Model file for the job. Use its own axes, mm. Face numbers are marked on the shaded views. A direction names the side the tool comes from. Give positions to 0.01 mm unless a question says otherwise; leave off trailing zeros. Loops run counter-clockwise (first coordinate to the right, second up) from the corner with the lowest first, then second, coordinate; pieces in that order, holes last. Notation, with made-up numbers: (-24.5, 78) -> (7.5, 78) arc R18 ccw to (7.5, 108) -> close; hole circle Ø10 at (-14, -29.75). An arc over 180 degrees is marked (long way). Use CSV: the item, a comma, the result in double quotes. Start each with the question number.
(1) Pull direction Y, two halves, no side cores. Call the marked faces 3, 4 and 5: pulls with the +Y half, pulls with the -Y half, needs draft (parallel to the pull), parting line crosses it, or undercut.
(2) Drill centre lines: probe 1 along X at (y, z) = (16, 2.25); probe 2 along X at (y, z) = (35.5, 6.75); probe 3 along Z at (x, y) = (23.5, 47). Where is each one in solid material? Low to high.
(3) Cut at B-B on y = 7. Write the cut outline in (x, z), then the cut area to 3 significant figures.
(4) Flat gauge pins, fed straight in: pin 1 (1.6 mm diameter, centred on x = 50, z = 4, fed in from +Y); pin 2 (0.8 mm diameter, centred on x = -18, z = 5.5, fed in from +Y); pin 3 (1.5 mm diameter, centred on x = 10.5, z = 6, fed in from -Y); pin 4 (1.2 mm diameter, centred on x = 35, y = 39.5, fed in from +Z). Where does each tip first touch, or does it go through?
(5) 3-axis set-ups, long thin cutter, end or side, ignore diameter. For the marked faces 1 and 2: which of +Z, -Z, +X, -X, +Y, -Y reach the whole face in a straight line?
(6) Cut at D-D on x = 43. Write the cut outline in (y, z).
(7) Cut at A-A on z = 4. State how many separate pieces and enclosed holes the cut face has, then the cut area to 3 significant figures.
(8) Cut at C-C on z = 9.75. Write the cut outline in (x, y).
Autodesk Inventor part; units mm, degrees
ref_plane "YZ Plane" through (0, 0, 0) normal (1, 0, 0) x (0, 1, 0)
ref_plane "XZ Plane" through (0, 0, 0) normal (0, 1, 0) x (-1, 0, 0)
ref_plane "XY Plane" through (0, 0, 0) normal (0, 0, 1) x (1, 0, 0)
sketch "Skizze1" plane through (0, 0, 0) normal (0, 0, 1) x (1, 0, 0)
  line L0 (-20.1131, -4) -> (51.8869, -4)
  line L1 (51.8869, -4) -> (51.8869, 40)
  line L2 (51.8869, 40) -> (-20.1131, 40)
  line L3 (-20.1131, 40) -> (-20.1131, -4)
  arc A0 (51.8869, 40) -> (-20.1131, 40) centre (15.8869, 5.3013) ccw
  line L4 (50.3869, -4) -> (50.3869, 40)
  line L5 (-18.6131, 40) -> (-18.6131, -4)
  arc A1 (50.3869, 40) -> (-18.6131, 40) centre (15.8869, 5.2581) ccw
  point P0 (0, 0)
  dimension "d0" = 72
  dimension "d1" = 44
  dimension "d2" = 50
  dimension "d3" = 1.5
  dimension "d4" = 1.5
extrude "Extrusion1" add sketch "Skizze1" along normal blind 2 contours L5 L2 L4 L0 | A1 L2
extrude "Extrusion2" add sketch "Skizze1" along normal blind 5 contours L3 L2 L5 L0 | A0 L2 A1 | L4 L2 L1 L0
sketch "Skizze2" plane through (0, 0, 2) normal (0, 0, 1) x (1, 0, 0)
  line L0 (50.3869, 40) -> (50.3869, -4)
  line L1 (50.3869, -4) -> (43.3869, -4)
  line L2 (-18.6131, 0) -> (-13.6131, 0)
  line L3 (-13.6131, 0) -> (-13.6131, -2)
  line L4 (-13.6131, -2) -> (-18.6131, -2)
  line L5 (-18.6131, -2) -> (-18.6131, 0)
  line L6 (45.3869, 0) -> (50.3869, 0)
  line L7 (50.3869, 0) -> (50.3869, -2)
  line L8 (50.3869, -2) -> (45.3869, -2)
  line L9 (45.3869, -2) -> (45.3869, 0)
  line L10 (-18.6131, -4) -> (50.3869, -4)
  circle A0 centre (-14.6131, 7) radius 2
  circle A1 centre (46.3869, 7) radius 2
  circle A2 centre (46.3869, 31) radius 2
  circle A3 centre (-14.6131, 31) radius 2
  line L11 (-18.6131, -4) -> (-18.6131, 40)
  circle A4 centre (-3.6131, 40) radius 1.05
  circle A5 centre (-3.6131, 40) radius 2
  circle A6 centre (35.3869, 40) radius 1.05
  circle A7 centre (35.3869, 40) radius 2
  line L12 (50.3869, 1) -> (48.8869, 1)
  line L13 (48.8869, 1) -> (48.8869, 36)
  line L14 (48.8869, 36) -> (50.3869, 36)
  line L15 (50.3869, 36) -> (50.3869, 1)
  line L16 (-18.6131, 36) -> (-17.1131, 36)
  line L17 (-17.1131, 36) -> (-17.1131, 1)
  line L18 (-17.1131, 1) -> (-18.6131, 1)
  line L19 (-18.6131, 1) -> (-18.6131, 36)
  point P0 (0, 0)
  point P1 (45.3869, -1)
  point P2 (-13.6131, -1)
  point P3 (-16.1131, -2)
  point P4 (49.6369, 1)
  point P5 (-17.8631, 1)
  dimension "d40" = 5
  dimension "d41" = 2
  dimension "d43" = 5
  dimension "d44" = 2
  dimension "d45" = 2
  dimension "d46" = 59
  dimension "d52" = 2
  dimension "d53" = 4
  dimension "d54" = 4
  dimension "d55" = 4
  dimension "d56" = 4
  dimension "d57" = 4
  dimension "d58" = 4
  dimension "d59" = 4
  dimension "d60" = 4
  dimension "d61" = 35
  dimension "d62" = 11
  dimension "d63" = 11
  dimension "d64" = 35
  dimension "d69" = 2.1
  dimension "d70" = 4
  dimension "d71" = 2.1
  dimension "d72" = 4
  dimension "d73" = 15
  dimension "d74" = 15
  dimension "d75" = 44
  dimension "d76" = 44
  dimension "d81" = 1.5
  dimension "d82" = 35
  dimension "d83" = 5
  dimension "d84" = 1.5
  dimension "d85" = 35
  dimension "d87" = 5
extrude "Extrusion7" add sketch "Skizze2" along normal blind 3 contours L5 L2 L3 L4 | L0 L8 L9 L6
extrude "Extrusion8" add sketch "Skizze2" along normal blind 11.5 contours A0 | A1 | A2 | A3
extrude "Extrusion9" add sketch "Skizze2" along normal blind 5 contours L11 L16 L17 L18 | L0 L12 L13 L14 | A5 | A7
extrude "Extrusion10" cut sketch "Skizze2" against normal up to next contours A4 | A6
properties part number "Spiel_Deckel"
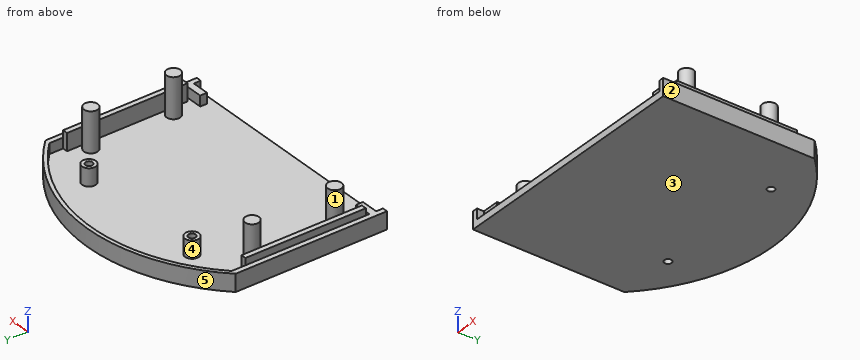
Check result:
1,face 3,"needs draft"
1,face 4,"undercut"
1,face 5,"pulls with the +Y half"
2,probe 1,"-20.11 to -17.11, 48.89 to 51.89"
2,probe 2,"-18.61 to -17.11, 48.89 to 50.39"
2,probe 3,"0 to 2"
3,outline,"(-20.11, 0) -> (51.89, 0) -> (51.89, 5) -> (50.39, 5) -> (50.39, 7) -> (48.89, 7) -> (48.89, 2) -> (48.39, 2) -> (48.39, 13.5) -> (44.39, 13.5) -> (44.39, 2) -> (-12.61, 2) -> (-12.61, 13.5) -> (-16.61, 13.5) -> (-16.61, 2) -> (-17.11, 2) -> (-17.11, 7) -> (-18.61, 7) -> (-18.61, 5) -> (-20.11, 5) -> close"
3,area,"260 mm²"
4,pin 1,"y = 42.59"
4,pin 2,"y = 36"
4,pin 3,"through"
4,pin 4,"z = 7"
5,face 1,"+Z"
5,face 2,"+Z, -Z, +X, +Y, -Y"
6,outline,"(-4, 0) -> (47.31, 0) -> (47.31, 5) -> (46.03, 5) -> (46.03, 2) -> (-4, 2) -> close"
7,separate pieces,"7"
7,enclosed holes,"2"
7,area,"410 mm²"
8,outline,"circle Ø4 at (-14.61, 7); circle Ø4 at (-14.61, 31); circle Ø4 at (46.39, 7); circle Ø4 at (46.39, 31)"
